from build123d import *

# Parameters (mm, degrees)
SKETCH1_R      = 4.25
EXTRUDE1_DEPTH = 6


with BuildPart() as part:
    # Sketch1 → Extrude1 (new body)
    with BuildSketch(Plane.XY):
        with BuildLine():
            Line((38, -55), (38, -30.119678905))
            ThreePointArc((38, -30.119678905), (37.772116295, -27.51495624), (37.095389312, -24.989376755))
            Line((37.095389312, -24.989376755), (33.987127064, -16.449496417))
            ThreePointArc((33.987127064, -16.449496417), (24.834222454, -4.521198893), (10.494811545, 0))
            Line((10.494811545, 0), (-10.494811545, 0))
            ThreePointArc((-10.494811545, 0), (-24.834222454, -4.521198893), (-33.987127064, -16.449496417))
            Line((-33.987127064, -16.449496417), (-37.095389312, -24.989376755))
            ThreePointArc((-37.095389312, -24.989376755), (-37.772116295, -27.51495624), (-38, -30.119678905))
            Line((-38, -30.119678905), (-38, -55))
            ThreePointArc((-38, -55), (-36.535533906, -58.535533906), (-33, -60))
            Line((-33, -60), (33, -60))
            ThreePointArc((33, -60), (36.535533906, -58.535533906), (38, -55))
        make_face()
        with Locations((-28, -32)):
            Circle(SKETCH1_R, mode=Mode.SUBTRACT)
        with Locations((28, -32)):
            Circle(SKETCH1_R, mode=Mode.SUBTRACT)
    extrude(amount=EXTRUDE1_DEPTH)


solid = part.part
Check sheet for the modelled part. Datum: model origin and axes. Units: mm. Round coordinates to 2 decimals unless told otherwise and drop trailing zeros. Order: outer loops, then holes, each group sorted by start corner. A loop starts at its lowest first (then second) coordinate and runs counter-clockwise, first axis right, second up.
(1) Cross-section at B-B, the plane y = -32. Enter the section's corners in (x, z).
(2) Cross-section at A-A, the plane z = 1.6. Enter the section's corners in (x, y).
(3) Scan lines: probe 1 along Y at (x, z) = (28, 1.6); probe 2 along Y at (x, z) = (-11, 1.55); probe 3 along Y at (x, z) = (-23.5, 5.35). Record each from-to range of solid material in increasing order.
(4) Go/stop test with a flat-tipped pin: P1, Ø7.5, axis at x = -28, y = -32, coming from the +Z side. Record where the tip stops, or that it passes through.
(5) Cross-section at C-C, the plane x = 28. Enter the section's corners in (y, z), and give its area (3 significant figures).
(6) Cross-section at D-D, the plane y = -8. Enter the section's corners in (x, z), and give its area (3 significant figures).
(7) Draft check along X on faces 1 (the flat face through (-38, -42, 3)), 2 (the cylindrical face through (37.78, -27.55, 2.96)), 3 (the flat face through (-1, -30, 6)), 4 (the cylindrical face through (24.63, -34.59, 2.96)). Enter one of: pulls with the +X half, pulls with the -X half, needs draft (parallel to the pull), parting line crosses it, or undercut.
Check sheet entries:
1. outline: (-38, 0) - (-32.25, 0) - (-32.25, 6) - (-38, 6) - close; (-23.75, 0) - (23.75, 0) - (23.75, 6) - (-23.75, 6) - close; (32.25, 0) - (38, 0) - (38, 6) - (32.25, 6) - close
2. outline: (-38, -55) arc R5 ccw to (-33, -60) - (33, -60) arc R5 ccw to (38, -55) - (38, -30.12) arc R15 ccw to (37.1, -24.99) - (33.99, -16.45) arc R25 ccw to (10.49, 0) - (-10.49, 0) arc R25 ccw to (-33.99, -16.45) - (-37.1, -24.99) arc R15 ccw to (-38, -30.12) - close; hole circle Ø8.5 at (-28, -32); hole circle Ø8.5 at (28, -32)
3. probe 1: y = -60 to -36.25, -27.75 to -7.15
3. probe 2: y = -60 to -0.01
3. probe 3: y = -60 to -3.65
4. P1: passes through
5. outline: (-60, 0) - (-36.25, 0) - (-36.25, 6) - (-60, 6) - close; (-27.75, 0) - (-7.15, 0) - (-7.15, 6) - (-27.75, 6) - close
5. area: 266 mm2
6. outline: (-28.83, 0) - (28.83, 0) - (28.83, 6) - (-28.83, 6) - close
6. area: 346 mm2
7. face 1: pulls with the -X half
7. face 2: pulls with the +X half
7. face 3: needs draft
7. face 4: undercut
